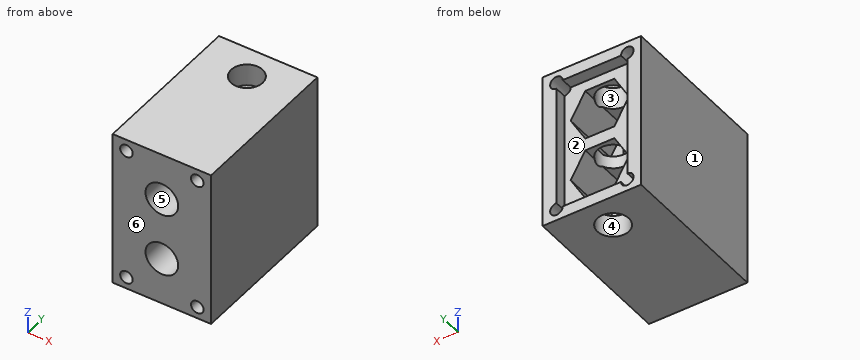
```python
from build123d import *

# Parameters (mm, degrees)
SKETCH1_W           = 25
SKETCH1_H           = 40
BOSS_EXTRUDE1_DEPTH = 40
SKETCH2_R           = 4
CUT_EXTRUDE1_DEPTH  = 58.933151131
SKETCH4_R           = 4.15
CUT_EXTRUDE2_DEPTH  = 47.435439053
CUT_EXTRUDE3_DEPTH  = 18
SKETCH6_R           = 1.6
CUT_EXTRUDE4_DEPTH  = 47.435439053
SKETCH7_W           = 18
SKETCH7_H           = 34
CUT_EXTRUDE5_DEPTH  = 3


with BuildPart() as part:
    # Sketch1 → Boss-Extrude1 (new body)
    with BuildSketch(Plane(origin=(0, 0, 0), x_dir=(1, 0, 0), z_dir=(0, 1, 0))):
        Rectangle(SKETCH1_W, SKETCH1_H)
    extrude(amount=BOSS_EXTRUDE1_DEPTH)

    # Sketch2 → Cut-Extrude1 (cut, through all)
    with BuildSketch(Plane.XY.offset(20)):
        with Locations((0, 32)):
            Circle(SKETCH2_R)
    extrude(amount=-CUT_EXTRUDE1_DEPTH, mode=Mode.SUBTRACT)

    # Sketch4 → Cut-Extrude2 (cut, through all)
    with BuildSketch(Plane(origin=(0, 40, 0), x_dir=(1, 0, 0), z_dir=(0, 1, 0))):
        with Locations(Location((0, -8, 0), (0, 0, 270))):
            Circle(SKETCH4_R)
        with Locations(Location((0, 8, 0), (0, 0, 270))):
            Circle(SKETCH4_R)
    extrude(amount=-CUT_EXTRUDE2_DEPTH, mode=Mode.SUBTRACT)

    # Sketch5 → Cut-Extrude3 (cut)
    with BuildSketch(Plane(origin=(0, 40, 0), x_dir=(1, 0, 0), z_dir=(0, 1, 0))):
        Polygon((-3.7, -14.408587988), (3.7, -14.408587988), (7.4, -8), (3.7, -1.591412012), (-3.7, -1.591412012), (-7.4, -8), align=None)
        Polygon((-3.7, 14.408587988), (-7.4, 8), (-3.7, 1.591412012), (3.7, 1.591412012), (7.4, 8), (3.7, 14.408587988), align=None)
    extrude(amount=-CUT_EXTRUDE3_DEPTH, mode=Mode.SUBTRACT)

    # Sketch6 → Cut-Extrude4 (cut, through all)
    with BuildSketch(Plane(origin=(0, 40, 0), x_dir=(1, 0, 0), z_dir=(0, 1, 0))):
        with Locations(Location((9, -17, 0), (0, 0, 270))):
            Circle(SKETCH6_R)
        with Locations(Location((-9, -17, 0), (0, 0, 270))):
            Circle(SKETCH6_R)
        with Locations(Location((-9, 17, 0), (0, 0, 270))):
            Circle(SKETCH6_R)
        with Locations(Location((9, 17, 0), (0, 0, 270))):
            Circle(SKETCH6_R)
    extrude(amount=-CUT_EXTRUDE4_DEPTH, mode=Mode.SUBTRACT)

    # Sketch7 → Cut-Extrude5 (cut)
    with BuildSketch(Plane(origin=(0, 40, 0), x_dir=(1, 0, 0), z_dir=(0, 1, 0))):
        Rectangle(SKETCH7_W, SKETCH7_H)
    extrude(amount=-CUT_EXTRUDE5_DEPTH, mode=Mode.SUBTRACT)


solid = part.part
```
Here's how the part is built. I have some questions about the finished solid (model axes, mm). Face numbers are marked on the shaded views. A direction names the side the tool comes from. Give positions to 0.01 mm unless a question says otherwise; leave off trailing zeros. Order: outer loops, then holes, each group sorted by start corner. A loop starts at its lowest first (then second) coordinate and runs counter-clockwise, first axis right, second up. Notation, with made-up numbers: M 23.5,77 L 66.5,77 A16 ccw 66.5,97 Z; hole C 29,69 d10. An arc over 180 degrees is marked long. Use a Markdown table: item, result. Add a question column.
1. Suppose I cut it at D-D (z = -4.5). List the corners of the cut face in (x, y) for me, and give its area (3 significant figures).
2. If we mould it in two halves opening along Y, with no side actions, what happens to the marked faces 3, 4, 5 and 6? For each: +Y half, -Y half, draft (parallel to the pull), parting line (faces both ways), or undercut.
3. On a 3-axis mill with a long thin cutter (end or side, diameter ignored), from which of +Z, -Z, +X, -X, +Y, -Y can I reach the whole of each face in a straight line? I mean the marked faces 1 and 2. Say none if no direction works.
4. Suppose I cut it at B-B (z = 1). List the corners of the cut face in (x, y) for me, and give its area (3 significant figures).
5. I need wall thicknesses on probe 1 along X at (y, z) = (26, -17); probe 2 along Z at (x, y) = (-9, 30.5); probe 3 along Z at (x, y) = (3, 25). Which ranges of each line are inside material? Lowest first, please. Write a range as from..to.
6. Suppose I cut it at A-A (y = 32). List the corners of the cut face in (x, z) for me.
7. For pin 1 Ø9 at (x, z) = (-1, -2.5) entering from +Y; pin 2 Ø6.5 at (x, z) = (1, -7.5) entering from +Y; pin 3 Ø5 at (x, z) = (0, 8) entering from -Y, each with a flat end and sliding along its axis, tell me the tip position at first contact or that it passes through.
8. Suppose I cut it at C-C (y = 9). List the corners of the cut face in (x, z) for me.
Results list:
| question | item | result |
|---|---|---|
| 1 | outline | M -12.5,0 L -2.23,0 L -2.23,22 L -5.38,22 L -5.38,37 L -9,37 L -9,40 L -12.5,40 Z; M 2.23,0 L 12.5,0 L 12.5,40 L 9,40 L 9,37 L 5.38,37 L 5.38,22 L 2.23,22 Z |
| 1 | area | 687 mm² |
| 2 | face 3 | undercut |
| 2 | face 4 | undercut |
| 2 | face 5 | draft |
| 2 | face 6 | -Y half |
| 3 | face 1 | +Z, -Z, -X, +Y, -Y |
| 3 | face 2 | +Y |
| 4 | outline | M -12.5,0 L 12.5,0 L 12.5,40 L 9,40 L 9,37 L -9,37 L -9,40 L -12.5,40 Z; hole C 0,32 d8 |
| 4 | area | 896 mm² |
| 5 | probe 1 | x = -12.5..-10.6, -7.4..7.4, 10.6..12.5 |
| 5 | probe 2 | z = -20..-18.6, -15.4..15.4, 18.6..20 |
| 5 | probe 3 | z = -20..-14.41, -1.59..1.59, 14.41..20 |
| 6 | outline | M -12.5,-20 L -4,-20 L -4,-13.89 L -7.4,-8 L -4,-2.11 L -4,2.11 L -7.4,8 L -4,13.89 L -4,20 L -12.5,20 Z; M 4,-20 L 12.5,-20 L 12.5,20 L 4,20 L 4,13.89 L 7.4,8 L 4,2.11 L 4,-2.11 L 7.4,-8 L 4,-13.89 Z; hole C -9,-17 d3.2; hole C -9,17 d3.2; hole C 9,-17 d3.2; hole C 9,17 d3.2 |
| 7 | pin 1 | stops at y = 37 |
| 7 | pin 2 | stops at y = 22 |
| 7 | pin 3 | passes through |
| 8 | outline | M -12.5,-20 L 12.5,-20 L 12.5,20 L -12.5,20 Z; hole C -9,-17 d3.2; hole C -9,17 d3.2; hole C 0,-8 d8.3; hole C 0,8 d8.3; hole C 9,-17 d3.2; hole C 9,17 d3.2 |
